Here's how the part is built. I have some questions about the finished solid (model axes, mm). A direction names the side the tool comes from. Give positions to 0.01 mm unless a question says otherwise; leave off trailing zeros. Order: outer loops, then holes, each group sorted by start corner. A loop starts at its lowest first (then second) coordinate and runs counter-clockwise, first axis right, second up.
from build123d import *

# Parameters (mm, degrees)
PAD_DEPTH       = 20
SKETCH001_R     = 2.25
POCKET_DEPTH    = 15.001
SKETCH002_R     = 5
POCKET001_DEPTH = 3


with BuildPart() as part:
    # Sketch → Pad (new body)
    with BuildSketch(Plane.XY):
        with BuildLine():
            ThreePointArc((-4.05, 0), (0, -4.05), (4.05, 0))
            Line((4.05, 0), (17.5, 0))
            Line((17.5, 0), (17.5, -15))
            Line((17.5, -15), (-17.5, -15))
            Line((-17.5, -15), (-17.5, 0))
            Line((-17.5, 0), (-4.05, 0))
        make_face()
    extrude(amount=PAD_DEPTH)

    # Sketch001 → Pocket (cut, through all)
    with BuildSketch(Plane.XZ.offset(15)):
        with Locations((-11, 10)):
            Circle(SKETCH001_R)
        with Locations((11, 10)):
            Circle(SKETCH001_R)
    extrude(amount=-POCKET_DEPTH, mode=Mode.SUBTRACT)

    # Sketch002 → Pocket001 (cut)
    with BuildSketch(Plane.XZ.offset(15)):
        with Locations((-11.052364, 10)):
            Circle(SKETCH002_R)
        with Locations((10.947636, 10)):
            Circle(SKETCH002_R)
    extrude(amount=-POCKET001_DEPTH, mode=Mode.SUBTRACT)


solid = part.part
Q1. I need wall thicknesses on L1, parallel to Z at x = -11, y = -5; L2, parallel to X at y = -13.75, z = 8.5; L3, parallel to Y at x = 14, z = 7.5. Which ranges of each line are inside material? Lowest first, please.
Filled sheet:
L1: z = 0 to 7.75, 12.25 to 20
L2: x = -17.5 to -15.82, -6.28 to 6.18, 15.72 to 17.5
L3: y = -12 to 0
Q2. I'm going to push a flat-ended pin straight in: P1, Ø3, axis at x = 13.5, z = 8.5, coming from the -Y side. Where does the tip first touch, or does it pass through?
Filled sheet:
P1: stops at y = -12
Q3. If we section it at C-C on x = 9.5: List the corners of the cut face in (y, z) for me.
Filled sheet:
outline: (-15, 0) - (0, 0) - (0, 8.32) - (-12, 8.32) - (-12, 5.21) - (-15, 5.21) - close; (-15, 14.79) - (-12, 14.79) - (-12, 11.68) - (0, 11.68) - (0, 20) - (-15, 20) - close
Q4. If we section it at A-A on z = 10: List the corners of the cut face in (x, y) for me.
Filled sheet:
outline: (-17.5, -15) - (-16.05, -15) - (-16.05, -12) - (-13.25, -12) - (-13.25, 0) - (-17.5, 0) - close; (-8.75, -12) - (-6.05, -12) - (-6.05, -15) - (5.95, -15) - (5.95, -12) - (8.75, -12) - (8.75, 0) - (4.05, 0) arc R4.05 cw to (-4.05, 0) - (-8.75, 0) - close; (13.25, -12) - (15.95, -12) - (15.95, -15) - (17.5, -15) - (17.5, 0) - (13.25, 0) - close
Q5. If we section it at D-D on y = -2.25: List the corners of the cut face in (x, z) for me, plus the area to 3 significant figures.
Filled sheet:
outline: (-17.5, 0) - (-3.37, 0) - (-3.37, 20) - (-17.5, 20) - close; (3.37, 0) - (17.5, 0) - (17.5, 20) - (3.37, 20) - close; hole circle Ø4.5 at (-11, 10); hole circle Ø4.5 at (11, 10)
area: 533 mm2
Q6. If we section it at B-B on y = -11.25: List the corners of the cut face in (x, z) for me, plus the area to 3 significant figures.
Filled sheet:
outline: (-17.5, 0) - (17.5, 0) - (17.5, 20) - (-17.5, 20) - close; hole circle Ø4.5 at (-11, 10); hole circle Ø4.5 at (11, 10)
area: 668 mm2
Q7. Thinking about a two-plate mould opening in X: for faces 1 (the face through (12, -12, 7.8)), 2 (the face through (10.7, 0, 7.6)), 3 (the face through (-17.5, -8, 10)), which applies, released by +X, released by -X, zero draft, split by the parting line, or undercut?
Filled sheet:
face 1: undercut
face 2: zero draft
face 3: released by -X
Q8. For faces 4 (the face through (0, -7, 0)), 5 (the face through (-10, -12, 7.8)), which set-ups out of +Z, -Z, +X, -X, +Y, -Y let a thin tool reach every point of the face, with its end or its side?
Filled sheet:
face 4: -Z, +X, -X, +Y, -Y
face 5: -Y
